from build123d import *

# Parameters (mm, degrees)
SKETCH1_R           = 3.175
BOSS_EXTRUDE2_DEPTH = 3.175


with BuildPart() as part:
    # Sketch1 → Boss-Extrude2 (new body)
    with BuildSketch(Plane.XY):
        with BuildLine():
            add(Edge.make_bspline(
                [(-459.058883104, 1020.90986665), (-454.410065073, 1009.258459074), (-444.447409236, 1016.856993556), (-434.4847534, 1024.455528037), (-444.447409236, 1032.054062519), (-454.410065073, 1039.652597001), (-459.058883104, 1028.001189425)],
                knots=[1.951262384, 1.951262384, 1.951262384, 3.792013448, 3.792013448, 5.632764512, 5.632764512, 7.473515577, 7.473515577, 7.473515577], degree=2, weights=[1, 0.60552134, 1, 0.60552134, 1, 0.60552134, 1]))
            Line((-459.058883104, 1028.001189425), (-459.74, 1028.001189425))
            Line((-459.74, 1028.001189425), (-459.74, 1075.255528037))
            ThreePointArc((-459.74, 1075.255528037), (-456.020256121, 1084.235784159), (-447.04, 1087.955528037))
            Line((-447.04, 1087.955528037), (-396.24, 1087.955528037))
            ThreePointArc((-396.24, 1087.955528037), (-387.259743879, 1084.235784159), (-383.54, 1075.255528037))
            Line((-383.54, 1075.255528037), (-383.54, 973.655528037))
            ThreePointArc((-383.54, 973.655528037), (-387.259743879, 964.675271916), (-396.24, 960.955528037))
            Line((-396.24, 960.955528037), (-447.04, 960.955528037))
            ThreePointArc((-447.04, 960.955528037), (-456.020256121, 964.675271916), (-459.74, 973.655528037))
            Line((-459.74, 973.655528037), (-459.74, 1020.90986665))
            Line((-459.74, 1020.90986665), (-459.058883104, 1020.90986665))
        make_face()
        with Locations((-421.64, 1024.455528037)):
            Circle(SKETCH1_R, mode=Mode.SUBTRACT)
        with Locations((-437.515, 986.355528037)):
            Circle(SKETCH1_R, mode=Mode.SUBTRACT)
        with Locations((-437.515, 1062.555528037)):
            Circle(SKETCH1_R, mode=Mode.SUBTRACT)
    extrude(amount=BOSS_EXTRUDE2_DEPTH)


solid = part.part
Design review of the part built by this model. Coordinates are the model's own, in mm. Coordinates: 2 decimals unless noted, no trailing zeros. Order: outer loops, then holes, each group sorted by start corner. A loop starts at its lowest first (then second) coordinate and runs counter-clockwise, first axis right, second up. Notation, with made-up numbers: (42, 61.5) -> (48, 61.5) arc R25 cw to (48, 89.5) -> close; hole circle Ø1 at (-24.75, 23.5). An arc over 180 degrees is marked (long way). One line per item, written item: value.
1) We need section A-A, the plane x = -421.64. Give the boundary of the cut face in (y, z) (3 decimals), then the cut area to 3 significant figures.
Output values:
outline: (960.956, 0) -> (1021.281, 0) -> (1021.281, 3.175) -> (960.956, 3.175) -> close; (1027.631, 0) -> (1087.956, 0) -> (1087.956, 3.175) -> (1027.631, 3.175) -> close
area: 383 mm2
2) To check wall thickness, follow probe 1 along Y at (x, z) = (-421.64, 1.75); probe 2 along X at (y, z) = (970, 0.6); probe 3 along Y at (x, z) = (-390.5, 2.95). State the ranges of each line that lie inside material, in increasing order. Write a range as [from, to].
Output values:
probe 1: y = [960.96, 1021.28], [1027.63, 1087.96]
probe 2: x = [-459.2, -384.08]
probe 3: y = [962.33, 1086.58]
3) Draft analysis for pull direction X (two halves, no side actions). For faces 1 (the face through (-455.921, 964.577, 1.565)), 2 (the face through (-387.359, 1084.334, 1.565)), 3 (the face through (-437.928, 989.504, 1.565)), 4 (the face through (-435.808, 1065.233, 1.565)), state which applies: +X half, -X half, draft (parallel to the pull), parting line (faces both ways), or undercut.
Output values:
face 1: -X half
face 2: +X half
face 3: undercut
face 4: undercut
4) We need section B-B, the plane z = 0.75. Count the separate pieces of the cut face and the enclosed holes in it, then the cut area to 3 significant figures.
Output values:
separate pieces: 1
enclosed holes: 3
area: 9,160 mm2
